Could you check a few things on this model? Use its own coordinates, in mm. Coordinates: 2 decimals unless noted, no trailing zeros. Order: outer loops, then holes, each group sorted by start corner. A loop starts at its lowest first (then second) coordinate and runs counter-clockwise, first axis right, second up. Notation, with made-up numbers: (4.5, 85.5) -> (49.5, 85.5) arc R23 ccw to (49.5, 108.5) -> close; hole circle Ø2 at (-11.75, -17). An arc over 180 degrees is marked (long way). Return JSON: item names as keys, results as strings. Group by question number.
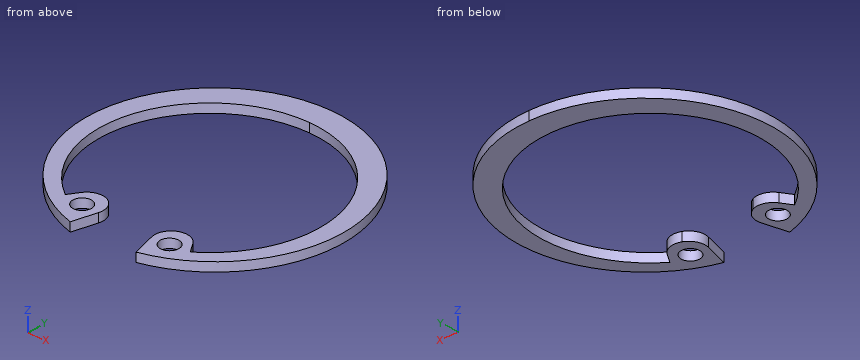
from build123d import *

# Parameters (mm, degrees)
SKETCH2_R           = 1.25
BOSS_EXTRUDE1_DEPTH = 1.2
FILLET1_R           = 2.197241


with BuildPart() as part:
    # Sketch2 → Boss-Extrude1 (new body)
    with BuildSketch(Plane.XY):
        with BuildLine():
            Line((6.518417516, -10.013392411), (8.436546126, -12.95996256))
            ThreePointArc((8.436546126, -12.95996256), (14.124578682, 3.619986092), (0, 14))
            Line((0, 14), (0, 17.2))
            ThreePointArc((0, 17.2), (17.052851616, 2.245050506), (4.451687576, -16.613924212))
            Line((4.451687576, -16.613924212), (3.092403424, -11.541006696))
            Line((3.092403424, -11.541006696), (6.518417516, -10.013392411))
        make_face()
        with Locations((5.904953543, -13.243168943)):
            Circle(SKETCH2_R, mode=Mode.SUBTRACT)
    extrude(amount=BOSS_EXTRUDE1_DEPTH)

    # Fillet1
    fillet1_edges = [part.edges().sort_by_distance(p)[0] for p in [
        (6.518417516, -10.013392411, 0.6),
        (3.092403424, -11.541006696, 0.6),
    ]]
    fillet(fillet1_edges, radius=FILLET1_R)

    # Mirror1: part across plane


with BuildPart() as part_1:
    add(part.part)
    add(part.part.mirror(Plane(origin=(0, 17.2, 1.2), x_dir=(0, 0, 1), z_dir=(1, 0, 0))))


solid = part_1.part
Q1. I want a section at B-B on x = -6. Please give me the cut outline in (y, z).
Q2. I need wall thicknesses on line 1 along Y through (x, z) = (-5.5, 0.1); line 2 along X through (y, z) = (-11, 0.15); line 3 along X through (y, z) = (-14, 0.7). Which ranges of each line are inside material? Lowest first, please. Write a range as from..to.
Q3. I want a section at D-D on z = 0.95. Please give me the cut outline in (x, y), and give its area (3 significant figures).
Q4. I want a section at A-A on y = 10. Please give me the cut outline in (x, z).
Q5. I'm going to push a flat-ended pin straight in: pin 1 Ø5 at (x, y) = (-6, -8.5) entering from -Z. Where does the tip first touch, or does it pass through?
Q6. I want a section at C-C on x = -10.5. Please give me the cut outline in (y, z).
Response values:
{
 "1": {"outline": "(-16.12, 0) -> (-14.49, 0) -> (-14.49, 1.2) -> (-16.12, 1.2) -> close; (-12, 0) -> (-10.61, 0) -> (-10.61, 1.2) -> (-12, 1.2) -> close; (12.73, 0) -> (16.12, 0) -> (16.12, 1.2) -> (12.73, 1.2) -> close"},
 "2": {"line 1": "y = -16.3..-14.43, -12.06..-10.6, 12.94..16.3", "line 2": "x = -13.22..-10.72, -6.98..-4.42, 4.42..6.98, 10.72..13.22", "line 3": "x = -9.99..-6.9, -4.91..-3.75, 3.75..4.91, 6.9..9.99"},
 "3": {"outline": "(-8.44, -12.96) arc R14.8 cw (long way) to (8.44, -12.96) -> (7.54, -11.59) arc R2.2 ccw to (3.58, -13.35) -> (4.45, -16.61) arc R17.2 ccw (long way) to (-4.45, -16.61) -> (-3.58, -13.35) arc R2.2 ccw to (-7.54, -11.59) -> close; hole circle Ø2.5 at (-5.9, -13.24); hole circle Ø2.5 at (5.9, -13.24)", "area": "247 mm²"},
 "4": {"outline": "(-13.99, 0) -> (-10.12, 0) -> (-10.12, 1.2) -> (-13.99, 1.2) -> close; (10.12, 0) -> (13.99, 0) -> (13.99, 1.2) -> (10.12, 1.2) -> close"},
 "5": {"pin 1": "stops at z = 0"},
 "6": {"outline": "(-13.62, 0) -> (-11.23, 0) -> (-11.23, 1.2) -> (-13.62, 1.2) -> close; (9.63, 0) -> (13.62, 0) -> (13.62, 1.2) -> (9.63, 1.2) -> close"}
}
